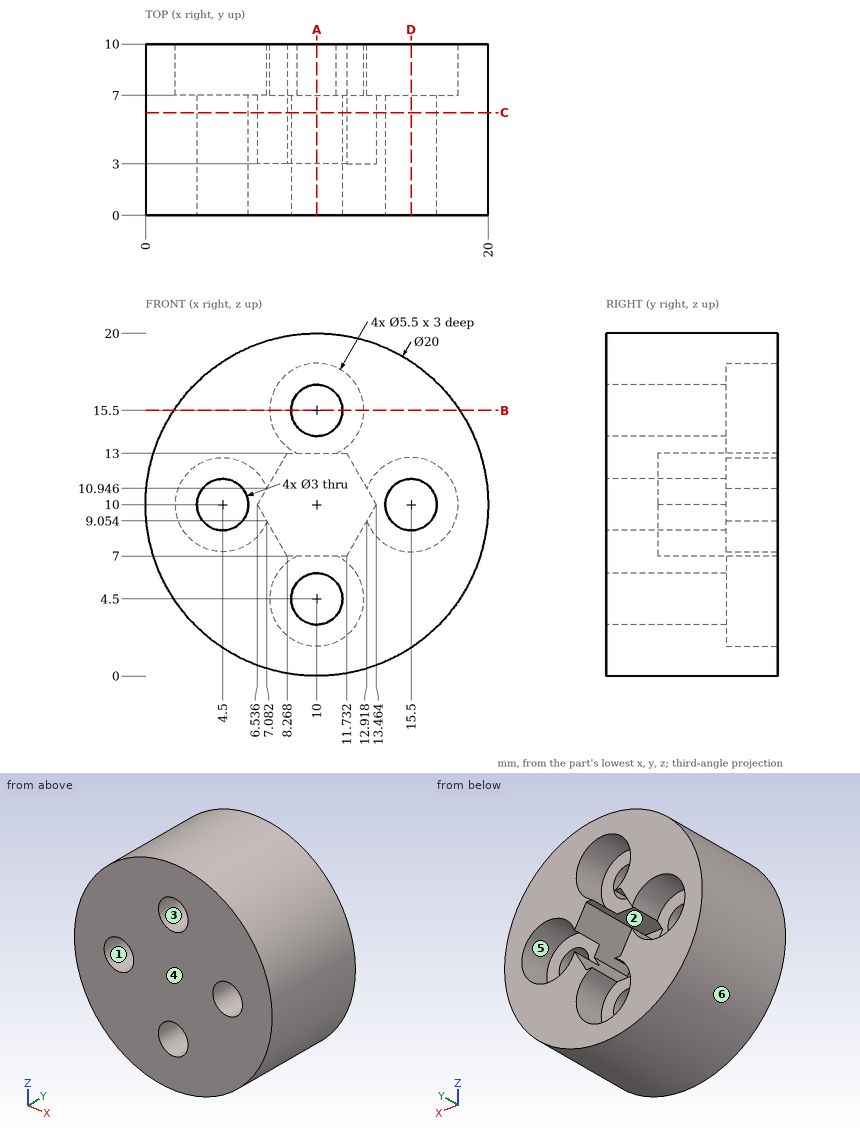
Here's the drawing with two shaded views (mm, measured from the low corner). I have some questions. A direction names the side the tool comes from. Give positions to 0.01 mm unless a question says otherwise; leave off trailing zeros. Write each loop counter-clockwise with the first axis right and the second up, starting at its lowest first coordinate (ties: lowest second). Pieces come first, ordered by that corner, then holes. Notation, with made-up numbers: (81.5, -20.75) -> (100.5, -20.75) arc R28 cw to (100.5, 6.25) -> close; hole circle Ø10 at (32, 58.5). An arc over 180 degrees is marked (long way). One line per item, written item: value.
Q1. Imagine slicing it at B-B on z = 15.5. Please give me the cut outline in (x, y).
Results found:
outline: (1.65, 0) -> (8.5, 0) -> (8.5, 7) -> (7.25, 7) -> (7.25, 10) -> (1.65, 10) -> close; (11.5, 0) -> (18.35, 0) -> (18.35, 10) -> (12.75, 10) -> (12.75, 7) -> (11.5, 7) -> close
Q2. Imagine slicing it at D-D on x = 15.5. Please give me the cut outline in (y, z).
Results found:
outline: (0, 1.65) -> (10, 1.65) -> (10, 7.25) -> (7, 7.25) -> (7, 8.5) -> (0, 8.5) -> close; (0, 11.5) -> (7, 11.5) -> (7, 12.75) -> (10, 12.75) -> (10, 18.35) -> (0, 18.35) -> close
Q3. We'd pull the mould along Z, two halves only. Please class the marked faces 3, 4, 5 and 6: +Z half, -Z half, draft (parallel to the pull), parting line (faces both ways), or undercut.
Results found:
face 3: undercut
face 4: draft
face 5: undercut
face 6: parting line
Q4. Please list where these lines run through material, in increasing order: line 1 (Z direction, x = 10, y = 4.75); line 2 (Z direction, x = 9.5, y = 5); line 3 (X direction, y = 7.75, z = 10). Write a range as [from, to].
Results found:
line 1: z = [0, 3], [6, 7], [13, 14], [17, 20]
line 2: z = [0.01, 3.09], [5.91, 7], [13, 14.09], [16.91, 19.99]
line 3: x = [0, 1.75], [18.25, 20]
Q5. For P1, Ø1, axis at x = 15.5, y = 5.5, coming from the +Z side; P2, Ø4, axis at x = 9, y = 6.5, coming from the +Z side; P3, Ø1, axis at x = 8, z = 5, coming from the +Y side; P4, Ø6, axis at x = 3, y = 5.5, coming from the -Z side (3 decimals), each with a flat end and sliding along its axis, tell me the tip position at first contact or that it passes through.
Results found:
P1: stops at z = 18.66
P2: stops at z = 20
P3: stops at y = 7
P4: stops at z = 0.835
Q6. Which directions (+Z, -Z, +X, -X, +Y, -Y) give clear straight access to the entire face, cutting with the end or side of a thin tool? Please do the marked faces 1 and 2.
Results found:
face 1: +Y, -Y
face 2: +Y
Q7. Imagine slicing it at A-A on x = 10. Please give me the cut outline in (y, z).
Results found:
outline: (0, 0) -> (10, 0) -> (10, 1.75) -> (7, 1.75) -> (7, 3) -> (0, 3) -> close; (0, 6) -> (7, 6) -> (7, 7) -> (3, 7) -> (3, 13) -> (7, 13) -> (7, 14) -> (0, 14) -> close; (0, 17) -> (7, 17) -> (7, 18.25) -> (10, 18.25) -> (10, 20) -> (0, 20) -> close
Q8. Imagine slicing it at C-C on y = 6. Please give me the cut outline in (x, z).
Results found:
outline: circle Ø20 at (10, 10); hole circle Ø3 at (4.5, 10); hole (6.54, 10) -> (8.27, 7) -> (11.73, 7) -> (13.46, 10) -> (11.73, 13) -> (8.27, 13) -> close; hole circle Ø3 at (10, 4.5); hole circle Ø3 at (10, 15.5); hole circle Ø3 at (15.5, 10)
